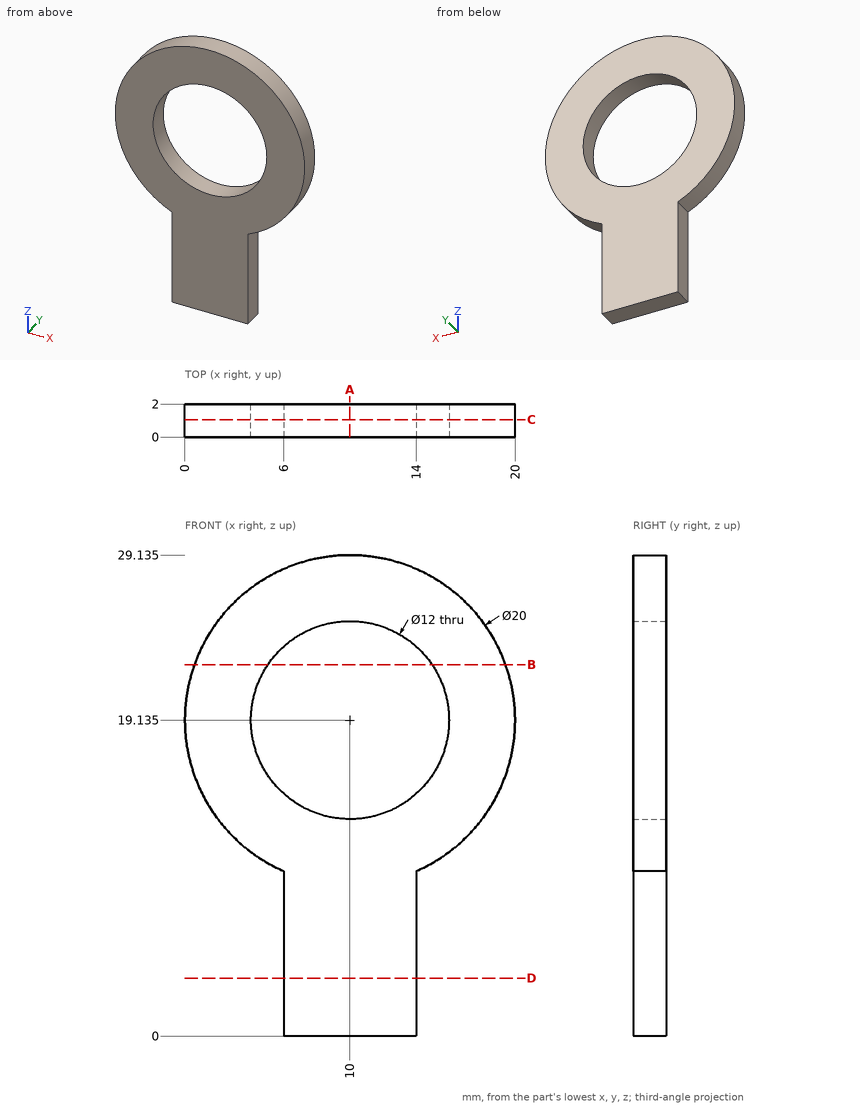
The figure shows three views and two pictorial views of one solid part (mm, origin at its lowest corner). Answer the questions. Give positions to 0.01 mm unless a question says otherwise; leave off trailing zeros. Write each loop counter-clockwise with the first axis right and the second up, starting at its lowest first coordinate (ties: lowest second). Pieces come first, ordered by that corner, then holes. Notation, with made-up numbers: M 25,85 L 39,85 A26 ccw 39,99 Z; hole C -15.5,81.25 d8. An arc over 180 degrees is marked long. One line per item, written item: value. Start each with the question number.
(1) Find section C-C (y = 1.05). Determine the outline of the cut face in (x, z) (3 decimals), plus the area to 3 significant figures.
(2) Find section A-A (x = 10). Determine the outline of the cut face in (y, z) (3 decimals), plus the area to 3 significant figures.
(3) Flat-ended cylindrical pins translate along their axes: pin 1 Ø1 at (y, z) = (0, 12) entering from -X; pin 2 Ø1 at (y, z) = (1, 6) entering from -X; pin 3 Ø9.5 at (x, z) = (10, 19.14) entering from +Y. Find the tip coordinate at first contact, or state that the pin passes through.
(4) Find the intervals of material crossed by line 1 (Z direction, x = 10, y = 0.55) (3 decimals); line 2 (Z direction, x = 2, y = 0.45) (1 decimal); line 3 (X direction, y = 0.95, z = 6.5), in increasing order.
(5) Find section D-D (z = 3.5). Determine the outline of the cut face in (x, y), plus the area to 3 significant figures.
(6) Find section B-B (z = 22.5). Determine the outline of the cut face in (x, y).
Results below:
1. outline: M 6,0 L 14,0 L 14,9.97 A10 ccw long 6,9.97 Z; hole C 10,19.135 d12
1. area: 276 mm^2
2. outline: M 0,0 L 2,0 L 2,13.135 L 0,13.135 Z; M 0,25.135 L 2,25.135 L 2,29.135 L 0,29.135 Z
2. area: 34.3 mm^2
3. pin 1: stops at x = 2.52
3. pin 2: stops at x = 6
3. pin 3: passes through
4. line 1: z = 0 to 13.135, 25.135 to 29.135
4. line 2: z = 13.1 to 25.1
4. line 3: x = 6 to 14
5. outline: M 6,0 L 14,0 L 14,2 L 6,2 Z
5. area: 16.0 mm^2
6. outline: M 0.58,0 L 5.03,0 L 5.03,2 L 0.58,2 Z; M 14.97,0 L 19.42,0 L 19.42,2 L 14.97,2 Z
